Geometry check sheet. Reference: the model listing, model coordinates, mm. Round coordinates to 2 decimals unless told otherwise and drop trailing zeros. Order: outer loops, then holes, each group sorted by start corner. A loop starts at its lowest first (then second) coordinate and runs counter-clockwise, first axis right, second up. Notation, with made-up numbers: (-7, -22) -> (7, -22) arc R9 ccw to (7, -12) -> close; hole circle Ø3 at (61.5, 60). An arc over 180 degrees is marked (long way). Use a Markdown table: item, result. Add a question column.
Item 1: Sectioned sample at C-C, the plane y = -103. Record the cut outline in (x, z), and give its area (3 significant figures).
Item 2: Gauge pin test, flat ends, axial feed: pin 1 Ø3 at (x, z) = (68.5, 0) entering from -Y; pin 2 Ø4.5 at (x, z) = (44.45, 0) entering from +Y; pin 3 Ø3 at (y, z) = (-158.5, -2) entering from +X; pin 4 Ø1 at (x, z) = (169.5, 1.5) entering from -Y. Record the tip position at first contact, or that the pin passes through.
Item 3: Sectioned sample at D-D, the plane x = 73.5. Record the cut outline in (y, z), and give its area (3 significant figures).
Item 4: Material ranges on probe 1 along Y at (x, z) = (12.7, 1.75); probe 2 along Z at (x, y) = (171.45, -7.25); probe 3 along X at (y, z) = (-175.5, 2.25), recorded low to high. Write a range as [from, to].
Item 5: Sectioned sample at A-A, the plane y = -177.8. Record the cut outline in (x, z).
Item 6: Sectioned sample at B-B, the plane x = 12.7. Record the cut outline in (y, z), and give its area (3 significant figures).
from build123d import *

# Parameters (mm, degrees)
BOSS_EXTRUDE1_DEPTH       = 4.7625
F_8_32_TAPPED_HOLE1_D     = 3.4544
F_8_32_TAPPED_HOLE1_DEPTH = 10.7188
F_8_32_TAPPED_HOLE1_TIP   = 1.037806461
CUT_EXTRUDE1_DEPTH        = 288.526008606
FILLET1_R                 = 6.35


with BuildPart() as part:
    # Sketch1 → Boss-Extrude1 (new, symmetric)
    with BuildSketch(Plane.XY):
        Polygon((0, -203.2), (0, 0), (203.2, 0), (203.2, -25.4), (25.4, -203.2), align=None)
    extrude(amount=BOSS_EXTRUDE1_DEPTH, both=True)

    # 8-32 Tapped Hole1
    with Locations(Plane(origin=(0, 0, 0), x_dir=(1, 0, 0), z_dir=(0, 1, 0))):
        with Locations((44.45, 0), (171.45, 0)):
            Hole(F_8_32_TAPPED_HOLE1_D / 2, depth=F_8_32_TAPPED_HOLE1_DEPTH)
            with Locations((0, 0, -(F_8_32_TAPPED_HOLE1_DEPTH + F_8_32_TAPPED_HOLE1_TIP / 2))):  # 118° drill point
                Cone(0, F_8_32_TAPPED_HOLE1_D / 2, F_8_32_TAPPED_HOLE1_TIP, mode=Mode.SUBTRACT)

    # Sketch6 → 1_4 Clearance Hole1 (revolve, cut)
    with BuildSketch(Plane(origin=(12.7, -177.8, 4.7625), x_dir=(0, -1, 0), z_dir=(1, 0, 0))):
        Polygon((0, 0), (0, 9.525), (4.0132, 9.525), (3.3782, 8.89), (3.3782, 0.635), (4.0132, 0), align=None)
    revolve(axis=Axis((12.7, -177.8, 11.1125), (0, 0, -1)), mode=Mode.SUBTRACT)

    # Sketch7 → Cut-Extrude1 (cut, through all)
    with BuildSketch(Plane.XY.offset(4.7625)):
        Polygon((25.4, -25.4), (25.4, -149.318463274), (149.318463274, -25.4), align=None)
    extrude(amount=-CUT_EXTRUDE1_DEPTH, mode=Mode.SUBTRACT)

    # Fillet1
    fillet1_edges = [part.edges().sort_by_distance(p)[0] for p in [
        (25.4, -25.4, 0),
        (149.318463274, -25.4, 0),
        (25.4, -149.318463274, 0),
    ]]
    fillet(fillet1_edges, radius=FILLET1_R)


solid = part.part
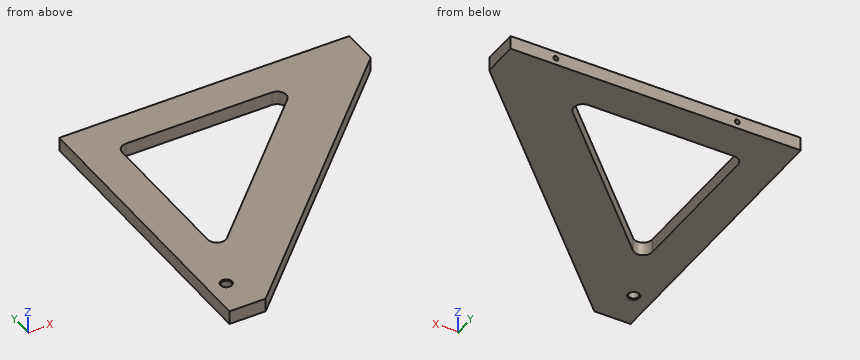
Found:
| question | item | result |
|---|---|---|
| 1 | outline | (0, -4.76) -> (25.4, -4.76) -> (25.4, 4.76) -> (0, 4.76) -> close; (71.72, -4.76) -> (125.6, -4.76) -> (125.6, 4.76) -> (71.72, 4.76) -> close |
| 1 | area | 755 mm2 |
| 2 | pin 1 | stops at y = -161.6 |
| 2 | pin 2 | stops at y = 0 |
| 2 | pin 3 | stops at x = 71.6 |
| 2 | pin 4 | stops at y = -59.6 |
| 3 | outline | (-155.1, -4.76) -> (-101.22, -4.76) -> (-101.22, 4.76) -> (-155.1, 4.76) -> close; (-25.4, -4.76) -> (0, -4.76) -> (0, 4.76) -> (-25.4, 4.76) -> close |
| 3 | area | 755 mm2 |
| 4 | probe 1 | y = [-203.2, -181.18], [-174.42, 0] |
| 4 | probe 2 | z = [-4.76, -1.73], [1.73, 4.76] |
| 4 | probe 3 | x = [0, 10.23], [15.17, 53.1] |
| 5 | outline | (0, -4.76) -> (8.69, -4.76) -> (9.32, -4.13) -> (9.32, 4.13) -> (8.69, 4.76) -> (0, 4.76) -> close; (16.08, -4.13) -> (16.71, -4.76) -> (50.8, -4.76) -> (50.8, 4.76) -> (16.71, 4.76) -> (16.08, 4.13) -> close |
| 6 | outline | (-203.2, -4.76) -> (-181.81, -4.76) -> (-181.18, -4.13) -> (-181.18, 4.13) -> (-181.81, 4.76) -> (-203.2, 4.76) -> close; (-174.42, -4.13) -> (-173.79, -4.76) -> (0, -4.76) -> (0, 4.76) -> (-173.79, 4.76) -> (-174.42, 4.13) -> close |
| 6 | area | 1,870 mm2 |
